```python
from build123d import *

# Parameters (mm, degrees)
ESBO_O9_W             = 3
ESBO_O9_H             = 5
CORTE_EXTRUS_O1_START = 1
CORTE_EXTRUS_O1_DEPTH = 1
PADR_OCIRCULAR2_COUNT = 3
CORTE_EXTRUS_O3_START = 0.9
CORTE_EXTRUS_O3_DEPTH = 0.9
PADR_OCIRCULAR4_COUNT = 3


with BuildPart() as part:
    # Esboço9 → Revolução1 (revolve)
    with BuildSketch(Plane.XY, mode=Mode.PRIVATE) as revolu_o1_sk:
        with Locations((8.75, 2.5)):
            Rectangle(ESBO_O9_W, ESBO_O9_H)
    revolve(revolu_o1_sk.sketch.rotate(Axis((0, -112.760074913, 0), (0, 1, 0)), 180), axis=Axis((0, -112.760074913, 0), (0, 1, 0)))

    # Esboço12 → Corte-extrusão1 (cut)
    with BuildSketch(Plane(origin=(0, 1.5, 0), x_dir=(1, 0, 0), z_dir=(0, 1, 0)).offset(CORTE_EXTRUS_O1_START)):
        with BuildLine():
            Line((0, 10.25), (0, 5.5))
            ThreePointArc((0, 5.5), (4.213244437, 3.535331853), (5.416442642, -0.955064977))
            Line((5.416442642, -0.955064977), (10.094279468, -1.779893821))
            ThreePointArc((10.094279468, -1.779893821), (7.851955542, 6.588572999), (0, 10.25))
        make_face()
    corte_extrus_o1 = extrude(amount=-CORTE_EXTRUS_O1_DEPTH, mode=Mode.SUBTRACT)

    # PadrãoCircular2: Corte-extrusão1 ×3 about axis
    padr_ocircular2_axis = Axis((0, 0, 0), (0, 1, 0))
    for i in range(1, PADR_OCIRCULAR2_COUNT):
        add(corte_extrus_o1.rotate(padr_ocircular2_axis, i * 360 / PADR_OCIRCULAR2_COUNT), mode=Mode.SUBTRACT)

    # Esboço13 → Corte-extrusão3 (cut)
    with BuildSketch(Plane(origin=(0, 3.3, 0), x_dir=(1, 0, 0), z_dir=(0, 1, 0)).offset(CORTE_EXTRUS_O3_START)):
        with BuildLine():
            Line((0, 0), (8.876760389, 5.125))
            ThreePointArc((8.876760389, 5.125), (9.631849363, -3.505706469), (3.505706469, -9.631849363))
            Line((3.505706469, -9.631849363), (0, 0))
        make_face()
    corte_extrus_o3 = extrude(amount=-CORTE_EXTRUS_O3_DEPTH, mode=Mode.SUBTRACT)

    # PadrãoCircular4: Corte-extrusão3 ×3 about axis
    padr_ocircular4_axis = Axis((0, 0, 0), (0, 1, 0))
    for i in range(1, PADR_OCIRCULAR4_COUNT):
        add(corte_extrus_o3.rotate(padr_ocircular4_axis, i * 360 / PADR_OCIRCULAR4_COUNT), mode=Mode.SUBTRACT)


solid = part.part
```
Read the model definition and answer for the solid it produces. Units are mm, in the model's axes. A direction names the side the tool comes from. Give positions to 0.01 mm unless a question says otherwise; leave off trailing zeros. Write each loop counter-clockwise with the first axis right and the second up, starting at its lowest first coordinate (ties: lowest second). Pieces come first, ordered by that corner, then holes. Notation, with made-up numbers: (-40, 67) -> (-35, 67) arc R16 ccw to (-35, 86) -> close; hole circle Ø8 at (-33, -24.75). An arc over 180 degrees is marked (long way). Answer as a JSON object with one key per item and string values.
1) Straight lines are drawn through the part: probe 1 along Y at (x, z) = (-4.5, 6.5); probe 2 along Z at (x, y) = (0, 3.1). For each, find the intervals that lie inside material, in ascending order. Write a range as from..to.
Findings below:
{"probe 1": "y = 0..1.5, 2.5..3.3, 4.2..5", "probe 2": "z = -10.25..-7.25, 7.25..10.25"}
2) A tool of negligible diameter and unlimited length cuts with its end or side. For faces 1 (the flat face through (8.596, 2.007, 1.516)), 2 (the flat face through (-7.56, 3.756, -4.365)), 3 (the flat face through (-5.611, 2.007, 6.687)), from which of +Z, -Z, +X, -X, +Y, -Y can it reach the whole face along a straight path? Write none if from no direction.
Findings below:
{"face 1": "-Z, +X", "face 2": "-Z", "face 3": "+Z, +X"}
3) Section B-B on y = 1.8 is taken. Write down the section's boundary in (x, z) (3 decimals).
Findings below:
{"outline": "(-8.877, 5.125) -> (-6.279, 3.625) arc R7.25 cw to (-4.66, 5.554) -> (-6.589, 7.852) arc R10.25 ccw to start; (-3.506, -9.632) arc R10.25 ccw to (0, -10.25) -> (0, -7.25) arc R7.25 cw to (-2.48, -6.813) -> close; (6.279, 3.625) arc R7.25 cw to (7.14, 1.259) -> (10.094, 1.78) arc R10.25 ccw to (8.877, 5.125) -> close"}
4) Flat-ended cylindrical pins translate along their axes: pin 1 Ø5 at (x, z) = (5.5, -4.5) entering from +Y; pin 2 Ø1 at (y, z) = (2.5, -4) entering from -X; pin 3 Ø1 at (y, z) = (3.5, 9) entering from -X. Find the tip coordinate at first contact, or state that the pin passes through.
Findings below:
{"pin 1": "stops at y = 5", "pin 2": "stops at x = -9.63", "pin 3": "stops at x = -5.67"}
5) Section C-C on z = 2.5 is taken. Write down the section's boundary in (x, y), then the cut area to 3 significant figures.
Findings below:
{"outline": "(-9.94, 0) -> (-6.81, 0) -> (-6.81, 1.5) -> (-9.94, 1.5) -> close; (-9.94, 2.5) -> (-6.81, 2.5) -> (-6.81, 3.3) -> (-9.94, 3.3) -> close; (-9.94, 4.2) -> (-6.81, 4.2) -> (-6.81, 5) -> (-9.94, 5) -> close; (6.81, 0) -> (9.94, 0) -> (9.94, 3.3) -> (6.81, 3.3) -> close; (6.81, 4.2) -> (9.94, 4.2) -> (9.94, 5) -> (6.81, 5) -> close", "area": "22.6 mm^2"}
6) For a pull along Y with two mould halves and no side action, classify faces 4 (the flat face through (0, 4, 9)), 5 (the flat face through (-7, 0, 2.4)) as pulls with the +Y half, pulls with the -Y half, needs draft (parallel to the pull), parting line crosses it, or undercut.
Findings below:
{"face 4": "undercut", "face 5": "pulls with the -Y half"}
7) Section A-A on z = 0 is taken. Write down the section's boundary in (x, y), then the cut area to 3 significant figures.
Findings below:
{"outline": "(-10.25, 0) -> (-7.25, 0) -> (-7.25, 1.5) -> (-10.25, 1.5) -> close; (-10.25, 2.5) -> (-7.25, 2.5) -> (-7.25, 3.3) -> (-10.25, 3.3) -> close; (-10.25, 4.2) -> (-7.25, 4.2) -> (-7.25, 5) -> (-10.25, 5) -> close; (7.25, 0) -> (10.25, 0) -> (10.25, 1.5) -> (7.25, 1.5) -> close; (7.25, 2.5) -> (10.25, 2.5) -> (10.25, 3.3) -> (7.25, 3.3) -> close; (7.25, 4.2) -> (10.25, 4.2) -> (10.25, 5) -> (7.25, 5) -> close", "area": "18.6 mm^2"}
8) Section D-D on x = 7.75 is taken. Write down the section's boundary in (y, z).
Findings below:
{"outline": "(0, -6.71) -> (1.5, -6.71) -> (1.5, 1.37) -> (2.5, 1.37) -> (2.5, -6.71) -> (5, -6.71) -> (5, 6.71) -> (4.2, 6.71) -> (4.2, -4.47) -> (3.3, -4.47) -> (3.3, 6.71) -> (2.5, 6.71) -> (2.5, 4.47) -> (1.5, 4.47) -> (1.5, 6.71) -> (0, 6.71) -> close"}
